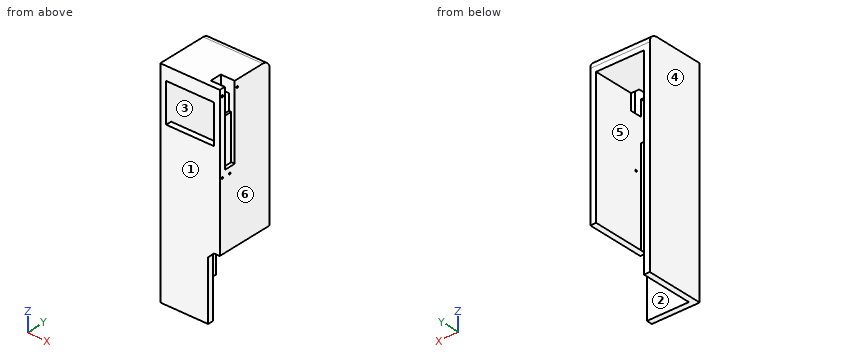
Solid Edge part; units mm, degrees
sketch "Sketch1" plane through (-117, 0, 0) normal (1, 0, 0) x (0, 1, 0)
  line L0 (117, 280.5) -> (117, 292)
  line L1 (117, 292) -> (67, 292)
  line L2 (67, 292) -> (67, 280.5)
  line L3 (67, 280.5) -> (117, 280.5)
extrude "Protrusion1" add sketch "Sketch1" along normal blind 102
fillet "Round_1" radius 7 1 edges at (-66, 117, 292)
sketch "Sketch2" plane through (-66, 92, 280.5) normal (0, 0, -1) x (1, 0, 0)
  line L0 (51, 25) -> (0, 25)
  line L1 (0, 25) -> (0, -25)
  line L2 (0, -25) -> (5, -25)
  line L3 (5, 20) -> (5, -25)
  line L4 (46, 20) -> (5, 20)
  line L5 (46, -25) -> (46, 20)
  line L6 (46, -25) -> (51, -25)
  line L7 (51, -25) -> (51, 25)
extrude "ExtrudedProtrusion_2" add sketch "Sketch2" along normal blind 171.5
sketch "Sketch3" plane through (-66, 67, 200.4979) normal (0, -1, 0) x (1, 0, 0)
  line L0 (5, 80.0021) -> (46, 80.0021)
  line L1 (46, 80.0021) -> (46, 46.5021)
  line L2 (46, 46.5021) -> (5, 46.5021)
  line L3 (5, 46.5021) -> (5, 80.0021)
extrude "Cutout1" cut sketch "Sketch3" against normal up to next
sketch "Sketch4" plane through (-15, 92, 200.4979) normal (1, 0, 0) x (0, 1, 0)
  line L0 (-10, 91.5021) -> (-10, 66.5021)
  line L1 (-10, 66.5021) -> (-20, 66.5021)
  line L2 (-20, 91.5021) -> (-20, 66.5021)
  line L3 (-20, 91.5021) -> (-10, 91.5021)
extrude "ExtrudedCutout_2" cut sketch "Sketch4" against normal blind 12
sketch "Sketch5" plane through (-15, 92, 200.4979) normal (1, 0, 0) x (0, 1, 0)
  line L0 (-10, 28.0021) -> (-10, 66.5021)
  line L1 (-10, 66.5021) -> (-20, 66.5021)
  line L2 (-20, 66.5021) -> (-20, 28.0021)
  line L3 (-20, 28.0021) -> (-10, 28.0021)
extrude "ExtrudedCutout_3" cut sketch "Sketch5" against normal blind 3
sketch "Sketch6" plane through (-15, 92, 200.4979) normal (1, 0, 0) x (0, 1, 0)
  circle A0 centre (-15, 23.0021) radius 0.8
extrude "Cutout2" cut sketch "Sketch6" against normal up to next
sketch "Sketch7" plane through (-15, 92, 200.4979) normal (1, 0, 0) x (0, 1, 0)
  circle A0 centre (-22.5, 85.5021) radius 0.8
  circle A1 centre (-7.5, 85.5021) radius 0.8
  circle A2 centre (-22.5, 23.0021) radius 0.8
extrude "ExtrudedCutout_5" cut sketch "Sketch7" against normal blind 6
sketch "Sketch8" plane through (-66, 67, 200.4979) normal (0, -1, 0) x (1, 0, 0)
  line L0 (46, -35.4979) -> (51, -35.4979)
  line L1 (51, -35.4979) -> (51, -91.4979)
  line L2 (51, -91.4979) -> (41.0042, -91.4979)
  line L3 (41.0042, -91.4979) -> (41.0042, -40.4937)
  line L4 (46, -35.4979) -> (41.0042, -40.4937)
extrude "Cutout3" cut sketch "Sketch8" against normal up to next
sketch "Sketch9" plane through (-117, 0, 0) normal (1, 0, 0) x (0, 1, 0)
  line L0 (117, 292) -> (67, 292)
  line L1 (67, 292) -> (67, 280.5)
  line L2 (67, 280.5) -> (117, 280.5)
  line L3 (117, 280.5) -> (117, 292)
extrude "ExtrudedCutout_7" cut sketch "Sketch9" along normal blind 51
Can you work these out from the model? Positions are in its coordinate system, mm. Face numbers are marked on the shaded views. A direction names the side the tool comes from. Give positions to 0.01 mm unless a question says otherwise; leave off trailing zeros. Write each loop counter-clockwise with the first axis right and the second up, starting at its lowest first coordinate (ties: lowest second). Pieces come first, ordered by that corner, then holes. Notation, with made-up numbers: (23, 32) -> (44, 32) arc R33 cw to (44, 63) -> close; hole circle Ø4 at (84.25, 2.25). An arc over 180 degrees is marked (long way). Answer as a JSON object with one key per item and string values. Group by question number.
Item 1: Suppose I cut it at A-A (x = -39). Please give me the cut outline in (y, z), plus the area to 3 significant figures.
Item 2: Please list where these lines run through material, in increasing order: line 1 (Y direction, x = -17.15, z = 223.5); line 2 (X direction, y = 108, z = 165.5); line 3 (Z direction, x = -16.55, y = 84.5). Write a range as [from, to].
Item 3: Suppose I cut it at B-B (y = 102). Please give me the cut outline in (x, z).
Item 4: We'd pull the mould along X, two halves only. Please class the marked faces 3, 4, 5 and 6: +X half, -X half, draft (parallel to the pull), parting line (faces both ways), or undercut.
Item 5: Suppose I cut it at D-D (z = 239). Please give me the cut outline in (x, y).
Item 6: For the marked faces 1 and 2, which set-ups out of +Z, -Z, +X, -X, +Y, -Y let a thin tool reach every point of the face, with its end or its side?
Item 7: Suppose I cut it at C-C (z = 168). Please give me the cut outline in (x, y), plus the area to 3 significant figures.
Item 8: I'm going to push flat-ended pins straight in: P1, Ø11, axis at y = 76, z = 287, coming from the +X side; P2, Ø0.5, axis at y = 70, z = 223.5, coming from the +X side; P3, Ø2.5, axis at x = -16.5, y = 78, coming from the +Z side; P4, Ø3, axis at x = -25, z = 210.5, coming from the +Y side. Where does each tip first touch, or does it pass through?
Findings:
{
 "1": {"outline": "(67, 109) -> (72, 109) -> (72, 247) -> (67, 247) -> close; (67, 280.5) -> (117, 280.5) -> (117, 285) arc R7 ccw to (110, 292) -> (67, 292) -> close", "area": "1,250 mm²"},
 "2": {"line 1": "y = [67, 68.7], [70.3, 76.2], [77.8, 117]", "line 2": "x = [-66, -61], [-20, -15]", "line 3": "z = [165, 285.2], [286.8, 292]"},
 "3": {"outline": "(-66, 109) -> (-61, 109) -> (-61, 280.5) -> (-20, 280.5) -> (-20, 165) -> (-15, 165) -> (-15, 292) -> (-66, 292) -> close"},
 "4": {"face 3": "undercut", "face 4": "-X half", "face 5": "undercut", "face 6": "+X half"},
 "5": {"outline": "(-66, 67) -> (-15, 67) -> (-15, 72) -> (-18, 72) -> (-18, 82) -> (-15, 82) -> (-15, 117) -> (-20, 117) -> (-20, 72) -> (-61, 72) -> (-61, 117) -> (-66, 117) -> close"},
 "6": {"face 1": "+Z, -Z, +X, -X, -Y", "face 2": "-Z, +Y"},
 "7": {"outline": "(-66, 67) -> (-15, 67) -> (-15, 117) -> (-20, 117) -> (-20, 72) -> (-61, 72) -> (-61, 117) -> (-66, 117) -> close", "area": "705 mm²"},
 "8": {"P1": "stops at x = -15", "P2": "stops at x = -21", "P3": "stops at z = 228.5", "P4": "stops at y = 72"}
}
